Read the model definition and answer for the solid it produces. Units are mm, in the model's axes. A direction names the side the tool comes from. Coordinates: 2 decimals unless noted, no trailing zeros. Loops run counter-clockwise (first coordinate to the right, second up) from the corner with the lowest first, then second, coordinate; pieces in that order, holes last. Notation, with made-up numbers: M -6.5,45.25 L 37.5,45.25 A16 cw 37.5,64.25 Z; hole C -29.5,-22 d3. An arc over 180 degrees is marked long. Put each result on its own line as item: value.
Autodesk Inventor part; units mm, degrees
ref_plane "Arbeitsebene2" through (-17.5, 40, 5.5) normal (0, -1, 0) x (1, 0, 0)
ref_plane "Arbeitsebene3" through (-17.5, -27.5, 0) normal (0, -1, 0) x (1, 0, 0)
ref_plane "YZ Plane" through (0, 0, 0) normal (1, 0, 0) x (0, 1, 0)
sketch "Skizze1" plane through (0, 0, 0) normal (0, 0, 1) x (1, 0, 0)
  line L0 (-17.5, 75) -> (17.5, 75)
  line L1 (17.5, 75) -> (17.5, -75)
  line L2 (17.5, -75) -> (-17.5, -75)
  line L3 (-17.5, -75) -> (-17.5, 75)
  line L4 (-17.5, 75) -> (17.5, -75) construction
  line L5 (17.5, 75) -> (-17.5, -75) construction
  point P0 (0, 0)
  dimension "d0" = 35
  dimension "d1" = 150
extrude "Extrusion1" add sketch "Skizze1" along normal blind 5.5
sketch "Skizze3" plane through (0, 0, 5.5) normal (0, 0, 1) x (1, 0, 0)
  line L0 (-17.5, 5) -> (17.5, 5)
  line L1 (17.5, 5) -> (17.5, 75)
  line L2 (17.5, 75) -> (-17.5, 75)
  line L3 (-17.5, 75) -> (-17.5, 5)
  line L4 (-17.5, 5) -> (17.5, 75) construction
  line L5 (17.5, 5) -> (-17.5, 75) construction
  line L6 (-17.5, 75) -> (-17.5, -75)
  line L7 (17.5, 75) -> (-17.5, 75)
  line L8 (17.5, -75) -> (17.5, 75)
  point P0 (0, 40)
  point P1 (-4.35, 75)
  point P2 (-17.5, 40)
  dimension "d8" = 70
extrude "Extrusion3" add sketch "Skizze3" along normal blind 20
ref_plane "Arbeitsebene2" through (-17.5, 40, 5.5) normal (0, -1, 0) x (1, 0, 0)
sketch "Skizze5" plane through (0, 0, 25.5) normal (0, 0, 1) x (1, 0, 0)
  line L0 (24.5, 40) -> (-24.5, 40)
  line L1 (0, 105) -> (0, -105)
  point P0 (0, 0)
  point P1 (0, 16)
  point P2 (0, 64)
  dimension "d23" = 24
  dimension "d24" = 24
hole "Bohrung2" at (0, 16, 25.5) at (0, 64, 25.5) direction (0, 0, -1) diameter 4.917 depth 16 tip angle 118
ref_plane "Arbeitsebene3" through (-17.5, -27.5, 0) normal (0, -1, 0) x (1, 0, 0)
sketch "Skizze6" plane through (0, 0, 5.5) normal (0, 0, 1) x (1, 0, 0)
  line L0 (0, 105) -> (0, -105)
  line L1 (-17.5, -75) -> (17.5, -75)
  point P0 (0, 0)
  point P1 (0, -55)
  point P2 (0, -15)
  dimension "d36" = 20
  dimension "d37" = 60
hole "Bohrung3" at (0, -55, 5.5) at (0, -15, 5.5) direction (0, 0, -1) diameter 9 end through all
properties part number "Adapterplatte_Vibrationsdaempfer"
1) Find section A-A, the plane y = -15. Write down the section's boundary in (x, z), plus the area to 3 significant figures.
Answer list:
outline: M -17.5,0 L -4.5,0 L -4.5,5.5 L -17.5,5.5 Z; M 4.5,0 L 17.5,0 L 17.5,5.5 L 4.5,5.5 Z
area: 143 mm^2
2) Given pin 1 Ø5 at (x, z) = (4, 12) entering from -Y; pin 2 Ø6 at (y, z) = (-18, 7) entering from +X; pin 3 Ø12 at (x, y) = (-4, -58) entering from +Z, each flat-ended and moving along its own axis, determine where each tip first touches the part or whether it passes through.
Answer list:
pin 1: stops at y = 5
pin 2: stops at x = 17.5
pin 3: stops at z = 5.5
3) Straight lines are drawn through the part: line 1 (Y direction, x = 0, z = 3.6); line 2 (Y direction, x = 0, z = 15.75); line 3 (X direction, y = 16, z = 19). For each, find the intervals that lie inside material, in ascending order. Write a range as [from, to].
Answer list:
line 1: y = [-75, -59.5], [-50.5, -19.5], [-10.5, 75]
line 2: y = [5, 13.54], [18.46, 61.54], [66.46, 75]
line 3: x = [-17.5, -2.46], [2.46, 17.5]
4) Find section B-B, the plane z = 2.75. Write down the section's boundary in (x, y), plus the area to 3 significant figures.
Answer list:
outline: M -17.5,-75 L 17.5,-75 L 17.5,75 L -17.5,75 Z; hole C 0,-55 d9; hole C 0,-15 d9
area: 5,120 mm^2
5) Find section C-C, the plane x = 14.5. Write down the section's boundary in (y, z), plus the area to 4 significant figures.
Answer list:
outline: M -75,0 L 75,0 L 75,25.5 L 5,25.5 L 5,5.5 L -75,5.5 Z
area: 2,225 mm^2
6) Which of the six approach directions +Z, -Z, +X, -X, +Y, -Y give full straight-line access (tool end or side, diameter ignored) to faces 4 (the cylindrical face through (-0.108, 18.456, 17.388)), 5 (the cylindrical face through (-0.198, -10.504, 2.712))?
Answer list:
face 4: +Z
face 5: +Z, -Z
7) Find section D-D, the plane z = 22. Write down the section's boundary in (x, y), plus the area to 3 significant figures.
Answer list:
outline: M -17.5,5 L 17.5,5 L 17.5,75 L -17.5,75 Z; hole C 0,16 d4.92; hole C 0,64 d4.92
area: 2,410 mm^2
8) Determine the mould class of faces 1 (the flat face through (0, -34, 5.5)), 2 (the cylindrical face through (0.94, 61.73, 17.39)), 3 (the flat face through (0, 5, 15)) for opening direction Y: released by +Y, released by -Y, zero draft, split by the parting line, or undercut.
Answer list:
face 1: zero draft
face 2: undercut
face 3: released by -Y
